CAD build for the part. Positions are in the model's coordinates, mm. Give positions to 0.01 mm unless a question says otherwise; leave off trailing zeros. Loops run counter-clockwise (first coordinate to the right, second up) from the corner with the lowest first, then second, coordinate; pieces in that order, holes last.
```python
from build123d import *

# Parameters (mm, degrees)
EXTRUDE_L_NGD_DEPTH = 1100
FILLET_KANTER_R     = 3


with BuildPart() as part:
    # Sketch3 → Extrude längd (new body)
    with BuildSketch(Plane(origin=(0, 0, 0), x_dir=(1, 0, 0), z_dir=(0, 1, 0))):
        Polygon((0, -80), (80, -80), (80, 0), (50, 0), (0, -50), align=None)
    extrude(amount=EXTRUDE_L_NGD_DEPTH)

    # Fillet kanter
    fillet_kanter_edges = [part.edges().sort_by_distance(p)[0] for p in [
        (80, 550, 80),
    ]]
    fillet(fillet_kanter_edges, radius=FILLET_KANTER_R)


solid = part.part
```
1. Saw through at C-C, the plane y = 553.5. List the corners of the cut face in (x, z), and give its area (3 significant figures).
Responses:
outline: (0, 50) - (50, 0) - (80, 0) - (80, 77) arc R3 ccw to (77, 80) - (0, 80) - close
area: 5,150 mm2
2. Probe line 1 along Z through (x, y) = (44.5, 661); line 2 along X through (y, z) = (181.5, 37); line 3 along X through (y, z) = (543, 45). List the from-to ranges inside material, lowest first.
Responses:
line 1: z = 5.5 to 80
line 2: x = 13 to 80
line 3: x = 5 to 80
3. Saw through at A-A, the plane x = 17.5. List the corners of the cut face in (y, z), and give its area (4 significant figures).
Responses:
outline: (0, 32.5) - (1100, 32.5) - (1100, 80) - (0, 80) - close
area: 52,250 mm2
4. Drop a flat-ended pin along its axis: pin 1 (4 mm diameter, centred on x = 16.5, y = 423.5, fed in from -Z). Give the stop position or say it passes through.
Responses:
pin 1: stops at z = 31.5
5. Saw through at B-B, the plane z = 15.5. List the corners of the cut face in (x, y).
Responses:
outline: (34.5, 0) - (80, 0) - (80, 1100) - (34.5, 1100) - close
